Autodesk Inventor part; units mm, degrees
ref_plane "YZ Plane" through (0, 0, 0) normal (1, 0, 0) x (0, 1, 0)
ref_plane "XZ Plane" through (0, 0, 0) normal (0, 1, 0) x (-1, 0, 0)
ref_plane "XY Plane" through (0, 0, 0) normal (0, 0, 1) x (1, 0, 0)
sketch "Sketch1" plane through (0, 0, 0) normal (0, 0, 1) x (1, 0, 0)
  line L0 (7, 7.5) -> (3, 7.5)
  line L1 (3, 7.5) -> (3, -7.5)
  line L2 (7, -7.5) -> (3, -7.5)
  line L3 (7, 7.5) -> (7, -7.5)
  circle A0 centre (5, -3.5) radius 1
  circle A1 centre (5, 3.5) radius 1
  line L4 (-3, 7.5) -> (-7, 7.5)
  line L5 (-7, -7.5) -> (-7, 7.5)
  line L6 (-3, -7.5) -> (-7, -7.5)
  line L7 (-3, -7.5) -> (-3, 7.5)
  circle A2 centre (-5, 3.5) radius 1
  circle A3 centre (-5, -3.5) radius 1
  point P0 (0, 0)
extrude "Extrusion1" add sketch "Sketch1" along normal blind 3
sketch "Sketch2" plane through (0, 0, 3) normal (0, 0, 1) x (1, 0, 0)
  line L0 (7, -7.5) -> (7, 7.5)
  line L1 (7, 7.5) -> (3, 7.5)
  line L2 (3, 7.5) -> (3, -7.5)
  line L3 (3, -7.5) -> (7, -7.5)
  circle A0 centre (5, -3.5) radius 1
  circle A1 centre (5, 3.5) radius 1
  line L4 (-3, -7.5) -> (-3, 7.5)
  line L5 (-3, 7.5) -> (-7, 7.5)
  line L6 (-7, 7.5) -> (-7, -7.5)
  line L7 (-7, -7.5) -> (-3, -7.5)
  circle A2 centre (-5, 3.5) radius 1
  circle A3 centre (-5, -3.5) radius 1
  line L8 (7, -7.5) -> (-7, -7.5)
  line L9 (-7, -7.5) -> (-7, 7.5)
  line L10 (-7, 7.5) -> (7, 7.5)
  line L11 (7, 7.5) -> (7, -7.5)
  point P0 (0, 0)
extrude "Extrusion2" add sketch "Sketch2" along normal blind 2
chamfer "Chamfer1" distance 2 angle 45 2 edges at (7, -7.5, 2.5) (-7, -7.5, 2.5)
fillet "Fillet1" radius 2 2 edges at (6, -6.5, 5) (-6, -6.5, 5)
properties part number "sub_arm_2"
The model under review builds one solid part; all positions refer to its coordinate system, in mm. A direction names the side the tool comes from. Coordinates: 2 decimals unless noted, no trailing zeros. Write each loop counter-clockwise with the first axis right and the second up, starting at its lowest first coordinate (ties: lowest second). Pieces come first, ordered by that corner, then holes. Notation, with made-up numbers: (57.25, -29) - (76.25, -29) arc R20 ccw to (76.25, 9) - close; hole circle Ø5 at (-33.75, -32). An arc over 180 degrees is marked (long way). Answer as a JSON object with one key per item and string values. Group by question number.
1. Machinability: for faces 1 (the face through (0, 0, 3)), 2 (the face through (7, 1, 2)), which of the approach directions +Z, -Z, +X, -X, +Y, -Y give a long, thin tool a straight path to every point of the face, cutting with its end or side? Answer none if there is none.
2. To check wall thickness, follow probe 1 along X at (y, z) = (-3.5, 2.2); probe 2 along X at (y, z) = (-1.75, 1.1); probe 3 along Y at (x, z) = (-5.25, 0.95). State the ranges of each line that lie inside material, in increasing order.
3. Add section C-C (y = 1.75). Give the boundary of the cut face in (x, z).
4. Add section B-B (y = 3.5). Give the boundary of the cut face in (x, z).
5. Add section A-A (z = 1.1). Give the boundary of the cut face in (x, y), plus the area to 3 significant figures.
6. Mouldability with a two-part tool opening along Y and no side actions: class faces 3 (the face through (5.42, -5.85, 4.65)), 4 (the face through (0, 7.5, 4)), 5 (the face through (-5.8, 4.1, 2.5)), 6 (the face through (-7, 1, 2)) as pulls with the +Y half, pulls with the -Y half, needs draft (parallel to the pull), parting line crosses it, or undercut.
7. Add section D-D (x = 5.5). Give the number of separate pieces and of enclosed holes in the cut face, plus the area to 3 significant figures.
Findings:
{
 "1": {"face 1": "-Z, +Y, -Y", "face 2": "+Z, -Z, +X, +Y, -Y"},
 "2": {"probe 1": "-7 to -6, -4 to -3, 3 to 4, 6 to 7", "probe 2": "-7 to -3, 3 to 7", "probe 3": "-7.25 to -4.47, -2.53 to 2.53, 4.47 to 7.5"},
 "3": {"outline": "(-7, 0) - (-3, 0) - (-3, 3) - (3, 3) - (3, 0) - (7, 0) - (7, 5) - (-7, 5) - close"},
 "4": {"outline": "(-7, 0) - (-6, 0) - (-6, 5) - (-7, 5) - close; (-4, 0) - (-3, 0) - (-3, 3) - (3, 3) - (3, 0) - (4, 0) - (4, 5) - (-4, 5) - close; (6, 0) - (7, 0) - (7, 5) - (6, 5) - close"},
 "5": {"outline": "(-7, -5.5) - (-5, -7.5) - (-3, -7.5) - (-3, 7.5) - (-7, 7.5) - close; (3, -7.5) - (5, -7.5) - (7, -5.5) - (7, 7.5) - (3, 7.5) - close; hole circle Ø2 at (-5, -3.5); hole circle Ø2 at (-5, 3.5); hole circle Ø2 at (5, -3.5); hole circle Ø2 at (5, 3.5)", "area": "103 mm²"},
 "6": {"face 3": "pulls with the -Y half", "face 4": "pulls with the +Y half", "face 5": "undercut", "face 6": "needs draft"},
 "7": {"separate pieces": "3", "enclosed holes": "0", "area": "54.0 mm²"}
}
